Source: CAD feature listing. Evaluate the final solid. Frame: model axes, mm. A direction names the side the tool comes from. Coordinates: 2 decimals unless noted, no trailing zeros. Write each loop counter-clockwise with the first axis right and the second up, starting at its lowest first coordinate (ties: lowest second). Pieces come first, ordered by that corner, then holes. Notation, with made-up numbers: (11.5, -35) -> (30.5, -35) arc R15 ccw to (30.5, -6) -> close; hole circle Ø7 at (42, 85). An arc over 180 degrees is marked (long way). Write item = value, one per line.
from build123d import *

# Parameters (mm, degrees)
SALIENTE_EXTRUIR1_DEPTH      = 200
CROQUIS2_R                   = 50
SALIENTE_EXTRUIR2_DEPTH      = 200
SALIENTE_EXTRUIR2_DEPTH_BACK = 400
CROQUIS3_W                   = 100
CROQUIS3_H                   = 100
CORTAR_EXTRUIR1_DEPTH        = 301
CROQUIS4_R                   = 52.5
CORTAR_EXTRUIR2_DEPTH        = 301
CHAFL_N1_SIZE                = 10


with BuildPart() as part:
    # Croquis1 → Saliente-Extruir1 (new body)
    with BuildSketch(Plane.XY):
        Polygon((-125, 100), (125, 100), (175, 100), (175, -100), (125, -100), (-125, -100), align=None)
    extrude(amount=SALIENTE_EXTRUIR1_DEPTH)

    # Croquis2 → Saliente-Extruir2 (add, two sides)
    with BuildSketch(Plane.XY.offset(200)) as saliente_extruir2_sk:
        Circle(CROQUIS2_R)
    extrude(amount=SALIENTE_EXTRUIR2_DEPTH)
    extrude(saliente_extruir2_sk.sketch, amount=-SALIENTE_EXTRUIR2_DEPTH_BACK)

    # Croquis3 → Cortar-Extruir1 (cut, through all)
    with BuildSketch(Plane(origin=(175, 0, 0), x_dir=(0, 0, -1), z_dir=(1, 0, 0))):
        with Locations((-100, 0)):
            Rectangle(CROQUIS3_W, CROQUIS3_H)
    extrude(amount=-CORTAR_EXTRUIR1_DEPTH, mode=Mode.SUBTRACT)

    # Croquis4 → Cortar-Extruir2 (cut, through all)
    with BuildSketch(Plane(origin=(175, 0, 0), x_dir=(0, 0, -1), z_dir=(1, 0, 0))):
        with Locations((-100, 0)):
            Circle(CROQUIS4_R)
    extrude(amount=-CORTAR_EXTRUIR2_DEPTH, mode=Mode.SUBTRACT)

    # Chaflán1
    chafl_n1_edges = [part.edges().sort_by_distance(p)[0] for p in [
        (175, 100, 100),
        (175, -100, 100),
        (25, 100, 200),
        (25, -100, 200),
        (25, -100, 0),
        (25, 100, 0),
        (175, 0, 0),
        (175, 0, 200),
    ]]
    chamfer(chafl_n1_edges, length=CHAFL_N1_SIZE)


solid = part.part
1) Cut plane B-B, the plane x = 0. Output: boundary loops of the cut face in (y, z).
Answer block:
outline = (-100, 10) -> (-90, 0) -> (-50, 0) -> (-50, -200) -> (50, -200) -> (50, 0) -> (90, 0) -> (100, 10) -> (100, 190) -> (90, 200) -> (50, 200) -> (50, 400) -> (-50, 400) -> (-50, 200) -> (-90, 200) -> (-100, 190) -> close; hole (-50, 50) -> (-16.01, 50) arc R52.5 ccw to (16.01, 50) -> (50, 50) -> (50, 83.99) arc R52.5 ccw to (50, 116.01) -> (50, 150) -> (16.01, 150) arc R52.5 ccw to (-16.01, 150) -> (-50, 150) -> (-50, 116.01) arc R52.5 ccw to (-50, 83.99) -> close
2) First-contact query: pin 1 Ø1 at (x, z) = (-32.5, -29.5) entering from +Y; pin 2 Ø10 at (x, y) = (-38, 41) entering from +Z; pin 3 Ø1.5 at (y, z) = (2, -9) entering from -X. Flat tips, straight axial feed; report the tip coordinate or a pass-through.
Answer block:
pin_1 = 38.42
pin_2 = 200
pin_3 = -49.98
3) Cut plane A-A, the plane y = 0. Output: boundary loops of the cut face in (x, z), and give its area (3 significant figures).
Answer block:
outline = (-125, 0) -> (-50, 0) -> (-50, -200) -> (50, -200) -> (50, 0) -> (165, 0) -> (175, 10) -> (175, 47.5) -> (-125, 47.5) -> close; (-125, 152.5) -> (175, 152.5) -> (175, 190) -> (165, 200) -> (50, 200) -> (50, 400) -> (-50, 400) -> (-50, 200) -> (-125, 200) -> close
area = 68,400 mm2
4) Material intervals for probe 1 along Z at (x, y) = (126.5, 24); probe 2 along Y at (x, z) = (160, 83); probe 3 along Z at (x, y) = (-16.5, 39), sorted ascending. Write a range as [from, to].
Answer block:
probe_1 = [0, 50], [150, 200]
probe_2 = [-100, -50], [50, 100]
probe_3 = [-200, 50], [150, 400]
5) Reachability of faces 1 (the flat face through (22, 100, 99)), 2 (the flat face through (27, 50, 133)) from +Z, -Z, +X, -X, +Y, -Y: full face, straight path, thin tool, end or side. Return the list, or none.
Answer block:
face_1 = +Z, -Z, +X, -X, +Y
face_2 = +X, -X
6) Cut plane C-C, the plane y = -69.5. Output: boundary loops of the cut face in (x, z), and give its area (3 significant figures).
Answer block:
outline = (-125, 0) -> (165, 0) -> (175, 10) -> (175, 190) -> (165, 200) -> (-125, 200) -> close
area = 59,900 mm2
7) Cut plane D-D, the plane x = -86. Output: boundary loops of the cut face in (y, z), and give its area (3 significant figures).
Answer block:
outline = (-100, 10) -> (-90, 0) -> (90, 0) -> (100, 10) -> (100, 190) -> (90, 200) -> (-90, 200) -> (-100, 190) -> close; hole (-50, 50) -> (-16.01, 50) arc R52.5 ccw to (16.01, 50) -> (50, 50) -> (50, 83.99) arc R52.5 ccw to (50, 116.01) -> (50, 150) -> (16.01, 150) arc R52.5 ccw to (-16.01, 150) -> (-50, 150) -> (-50, 116.01) arc R52.5 ccw to (-50, 83.99) -> close
area = 29,600 mm2
8) Pull-direction query (Z, two-part tool) for faces 3 (the flat face through (54, 1, 200)), 4 (the flat face through (27, -33, 50)), 5 (the cylindrical face through (47.69, 15.02, -98.6)), 6 (the cylindrical face through (27.1, -52.5, 100.2)); classes: +Z half, -Z half, draft (parallel to the pull), parting line (faces both ways), or undercut.
Answer block:
face_3 = +Z half
face_4 = undercut
face_5 = draft
face_6 = undercut
